Part model, mm, in its own coordinate system. Round coordinates to 2 decimals unless told otherwise and drop trailing zeros. Order: outer loops, then holes, each group sorted by start corner. A loop starts at its lowest first (then second) coordinate and runs counter-clockwise, first axis right, second up. Notation, with made-up numbers: (46.25, 47.5) - (97.25, 47.5) arc R17 cw to (97.25, 66.5) - close; hole circle Ø1 at (-35.75, 30.25). An arc over 180 degrees is marked (long way). Answer as a JSON object with one key per item and string values.
```python
from build123d import *

# Parameters (mm, degrees)
SKETCH1_R           = 1.5
BOSS_EXTRUDE1_DEPTH = 6
CUT_SWEEP1_PITCH    = 0.5
SKETCH5_W           = 11.492043773
SKETCH5_H           = 0.85
CUT_EXTRUDE1_DEPTH  = 2


with BuildPart() as part:
    # Sketch1 → Boss-Extrude1 (new body)
    with BuildSketch(Plane.XY):
        Circle(SKETCH1_R)
    extrude(amount=BOSS_EXTRUDE1_DEPTH)

    # Cut-Sweep1: arcs per turn and ends read off the stored shape
    # Cut-Sweep1: the profile of Sketch3 screwed along a right-hand helix through 7 turns, 6 arcs to a turn; built about Z, then put on its axis
    cut_sweep1_z = Axis((0, 0, 0), (0, 0, 1))
    cut_sweep1_corners = [(1.094191853, 0.001044043, -0.519679739), (1.509884047, -0.011670473, -0.280016765), (1.509884047, 0.013758558, -0.759342713)]
    with BuildLine(mode=Mode.PRIVATE) as cut_sweep1_profile:
        Line(cut_sweep1_corners[0], cut_sweep1_corners[1])
        Line(cut_sweep1_corners[1], cut_sweep1_corners[2])
        Line(cut_sweep1_corners[2], cut_sweep1_corners[0])
    cut_sweep1_cap = Face(cut_sweep1_profile.wire())
    cut_sweep1_turn_angles = [0, 30, 60, 90, 120, 150, 180, 210, 240, 270, 300, 330, 360]
    cut_sweep1_turn_weights = [1, 0.8660254037844387, 1, 0.8660254037844387, 1, 0.8660254037844387, 1, 0.8660254037844387, 1, 0.8660254037844387, 1, 0.8660254037844387, 1]
    cut_sweep1_turn_rails = [Edge.make_bspline([Vector(p[0], p[1], 0).rotate(cut_sweep1_z, cut_sweep1_turn_angles[k]) / cut_sweep1_turn_weights[k] + Vector(0, 0, p[2] + CUT_SWEEP1_PITCH * cut_sweep1_turn_angles[k] / 360) for k in range(13)], [0, 0, 0, 1, 1, 2, 2, 3, 3, 4, 4, 5, 5, 6, 6, 6], 2, cut_sweep1_turn_weights) for p in cut_sweep1_corners]
    cut_sweep1_turn_sides = [Face.make_surface_from_curves(cut_sweep1_turn_rails[p[0]], cut_sweep1_turn_rails[p[1]]) for p in [(0, 1), (1, 2), (2, 0)]]
    cut_sweep1 = Plane(origin=(0, 0, 6), x_dir=(-1, 0, 0), z_dir=(0, 0, -1)) * Solid(Shell([*[p.moved(Location((0, 0, CUT_SWEEP1_PITCH * i))) for i in range(7) for p in cut_sweep1_turn_sides], cut_sweep1_cap, cut_sweep1_cap.rotate(cut_sweep1_z, 2520).moved(Location((0, 0, CUT_SWEEP1_PITCH * 2520 / 360)))]))
    add(cut_sweep1, mode=Mode.SUBTRACT)

    # Sketch4 → Revolve1 (revolve)
    with BuildSketch(Plane(origin=(0, 0, 0), x_dir=(0, 0, -1), z_dir=(1, 0, 0)), mode=Mode.PRIVATE) as revolve1_sk:
        with BuildLine():
            Line((0, -3.110484298), (0, 0))
            Line((0, 0), (1.827405733, 0))
            add(Edge.make_bspline(
                [(1.827405733, 0), (1.614806924, -1.993581121), (0, -3.110484298)],
                knots=[0, 0, 0, 1, 1, 1], degree=2))
        make_face()
    revolve(revolve1_sk.sketch.rotate(Axis((0, 0, 0), (0, 0, -1)), 89.565814591), axis=Axis((0, 0, 0), (0, 0, -1)))

    # Sketch5 → Cut-Extrude1 (cut)
    with BuildSketch(Plane.XY.offset(-0.396562646)):
        with Locations((0.364356631, 0)):
            Rectangle(SKETCH5_W, SKETCH5_H)
    extrude(amount=-CUT_EXTRUDE1_DEPTH, mode=Mode.SUBTRACT)


solid = part.part
```
Item 1: Drop flat-ended pins along their axis: P1, Ø0.7, axis at x = -1, y = 0, coming from the -Z side; P2, Ø2, axis at x = -2.5, y = 1.5, coming from the +Z side; P3, Ø1.5, axis at y = 1.5, z = 5, coming from the -X side. Give the stop position or say it passes through.
Taken from the geometry:
{"P1": "z = -0.4", "P2": "z = 0", "P3": "x = -1.28"}
Item 2: Probe L1, parallel to Y at x = -0.5, z = -1.25 (3 decimals); L2, parallel to Z at x = 2.25, y = 0; L3, parallel to Y at x = 1, z = 3.5. List the from-to ranges inside material, lowest first. Write a range as from..to.
Taken from the geometry:
{"L1": "-1.728..-0.425, 0.425..1.728", "L2": "-0.4..0", "L3": "-1.05..0.96"}
Item 3: Two-plate mould, pull along Y, no slides. Class faces 1 (the flat face through (0, -0.425, -1)), 2 (the flat face through (0, 0, 6)): pulls with the +Y half, pulls with the -Y half, needs draft (parallel to the pull), parting line crosses it, or undercut.
Taken from the geometry:
{"face 1": "undercut", "face 2": "needs draft"}
Item 4: Cut at A-A (z = 1.25). Write the cut outline in (x, y).
Taken from the geometry:
{"outline": "circle Ø3 at (0, 0)"}
